The model under review builds one solid part; all positions refer to its coordinate system, in mm. A direction names the side the tool comes from. Coordinates: 2 decimals unless noted, no trailing zeros. Write each loop counter-clockwise with the first axis right and the second up, starting at its lowest first coordinate (ties: lowest second). Pieces come first, ordered by that corner, then holes. Notation, with made-up numbers: (-11, 82) -> (-6, 82) arc R9 cw to (-6, 94) -> close; hole circle Ø1 at (-24.75, 52). An arc over 180 degrees is marked (long way). Write each question's results on one line, items separated by ' | '.
```python
from build123d import *

# Parameters (mm, degrees)
SKETCH1_W           = 7.25
SKETCH1_H           = 7.25
BOSS_EXTRUDE1_DEPTH = 4
SKETCH3_W           = 5.1
SKETCH3_H           = 5.1
BOSS_EXTRUDE2_DEPTH = 1
SKETCH4_W           = 4.1
SKETCH4_H           = 4.1
CUT_EXTRUDE2_DEPTH  = 4
FILLET1_R           = 0.5


with BuildPart() as part:
    # Sketch1 → Boss-Extrude1 (new body)
    with BuildSketch(Plane(origin=(0, 0, 0), x_dir=(1, 0, 0), z_dir=(0, 1, 0))):
        Rectangle(SKETCH1_W, SKETCH1_H)
    extrude(amount=BOSS_EXTRUDE1_DEPTH)

    # Sketch3 → Boss-Extrude2 (add)
    with BuildSketch(Plane(origin=(0, 4, 0), x_dir=(1, 0, 0), z_dir=(0, 1, 0))):
        Rectangle(SKETCH3_W, SKETCH3_H)
    extrude(amount=BOSS_EXTRUDE2_DEPTH)

    # Sketch4 → Cut-Extrude2 (cut)
    with BuildSketch(Plane(origin=(0, 5, 0), x_dir=(1, 0, 0), z_dir=(0, 1, 0))):
        Rectangle(SKETCH4_W, SKETCH4_H)
    extrude(amount=-CUT_EXTRUDE2_DEPTH, mode=Mode.SUBTRACT)

    # Fillet1
    fillet1_edges = [part.edges().sort_by_distance(p)[0] for p in [
        (0, 0, 3.625),
        (-3.625, 0, 0),
        (0, 0, -3.625),
        (3.625, 0, 0),
        (3.625, 2, 3.625),
        (-3.625, 2, 3.625),
        (-3.625, 2, -3.625),
        (3.625, 2, -3.625),
    ]]
    fillet(fillet1_edges, radius=FILLET1_R)


solid = part.part
```
Q1. For line 1 (Z direction, x = 0, y = 1.8) (3 decimals); line 2 (X direction, y = 4.6, z = -2), list the stretches that pass through material, from the lowest coordinate up. Write a range as from..to.
Solution:
line 1: -3.625..-2.05, 2.05..3.625 | line 2: -2.55..-2.05, 2.05..2.55
Q2. Add section A-A (y = 1.65). Write out the cut boundary in (x, z) (3 decimals), plus the area to 3 significant figures.
Solution:
outline: (-3.625, -3.125) arc R0.5 ccw to (-3.125, -3.625) -> (3.125, -3.625) arc R0.5 ccw to (3.625, -3.125) -> (3.625, 3.125) arc R0.5 ccw to (3.125, 3.625) -> (-3.125, 3.625) arc R0.5 ccw to (-3.625, 3.125) -> close; hole (-2.05, -2.05) -> (2.05, -2.05) -> (2.05, 2.05) -> (-2.05, 2.05) -> close | area: 35.5 mm²
Q3. Add section B-B (x = -1.25). Write out the cut boundary in (y, z) (3 decimals), plus the area to 3 significant figures.
Solution:
outline: (0, -3.125) arc R0.5 ccw to (0.5, -3.625) -> (4, -3.625) -> (4, -2.55) -> (5, -2.55) -> (5, -2.05) -> (1, -2.05) -> (1, 2.05) -> (5, 2.05) -> (5, 2.55) -> (4, 2.55) -> (4, 3.625) -> (0.5, 3.625) arc R0.5 ccw to (0, 3.125) -> close | area: 17.6 mm²
Q4. Add section C-C (z = 0.75). Write out the cut boundary in (x, y) (3 decimals).
Solution:
outline: (-3.625, 0.5) arc R0.5 ccw to (-3.125, 0) -> (3.125, 0) arc R0.5 ccw to (3.625, 0.5) -> (3.625, 4) -> (2.55, 4) -> (2.55, 5) -> (2.05, 5) -> (2.05, 1) -> (-2.05, 1) -> (-2.05, 5) -> (-2.55, 5) -> (-2.55, 4) -> (-3.625, 4) -> close
Q5. Machinability: for faces 5 (the flat face through (2.55, 4.5, 0)), 6 (the flat face through (0, 4.5, -2.55)), 7 (the flat face through (-2.05, 3, 0)), which of the approach directions +Z, -Z, +X, -X, +Y, -Y give a long, thin tool a straight path to every point of the face, cutting with its end or side? Answer none if there is none.
Solution:
face 5: +Z, -Z, +X, +Y | face 6: -Z, +X, -X, +Y | face 7: +Y
Q6. Draft analysis for pull direction X (two halves, no side actions). For faces 1 (the flat face through (0, 3, 2.05)), 2 (the flat face through (0, 2, 3.625)), 3 (the flat face through (-3.625, 2, 0)), 4 (the flat face through (2.05, 3, 0)), state which applies: pulls with the +X half, pulls with the -X half, needs draft (parallel to the pull), parting line crosses it, or undercut.
Solution:
face 1: undercut | face 2: needs draft | face 3: pulls with the -X half | face 4: undercut
Q7. Clearance check with flat-ended pins moving along their axes: P1, Ø0.8, axis at y = 4.5, z = -1, coming from the -X side; P2, Ø2, axis at x = 0.5, z = 0.5, coming from the +Y side; P3, Ø1.1, axis at y = 4.5, z = 0, coming from the +X side (3 decimals). State where each tip first meets the part, or that it passes through.
Solution:
P1: x = -2.55 | P2: y = 1 | P3: x = 3.625
Q8. Add section D-D (y = 4.6). Write out the cut boundary in (x, z), plus the area to 3 significant figures.
Solution:
outline: (-2.55, -2.55) -> (2.55, -2.55) -> (2.55, 2.55) -> (-2.55, 2.55) -> close; hole (-2.05, -2.05) -> (2.05, -2.05) -> (2.05, 2.05) -> (-2.05, 2.05) -> close | area: 9.20 mm²
